```python
from build123d import *

# Parameters (mm, degrees)
F0_R     = 90.4875
F1_DEPTH = 63.5


with BuildPart() as f1:
    # F0 (on Top) → F1 (new body)
    with BuildSketch(Plane.XY):
        Circle(F0_R)
        with BuildLine():
            ThreePointArc((-6.35, -88.672924), (-76.989658, -44.45), (-79.968005, 38.837201))
            Line((-79.968005, 38.837201), (-77.415028, 37.363239))
            Line((-77.415028, 37.363239), (-74.240028, 42.8625))
            Line((-74.240028, 42.8625), (-71.065028, 48.361761))
            Line((-71.065028, 48.361761), (-73.618005, 49.835723))
            ThreePointArc((-73.618005, 49.835723), (0, 88.9), (73.618005, 49.835723))
            Line((73.618005, 49.835723), (71.065028, 48.361761))
            Line((71.065028, 48.361761), (74.240028, 42.8625))
            Line((74.240028, 42.8625), (77.415028, 37.363239))
            Line((77.415028, 37.363239), (79.968005, 38.837201))
            ThreePointArc((79.968005, 38.837201), (76.989658, -44.45), (6.35, -88.672924))
            Line((6.35, -88.672924), (6.35, -85.725))
            Line((6.35, -85.725), (0, -85.725))
            Line((0, -85.725), (-6.35, -85.725))
            Line((-6.35, -85.725), (-6.35, -88.672924))
        make_face(mode=Mode.SUBTRACT)
    extrude(amount=F1_DEPTH)


solid = f1.part
```
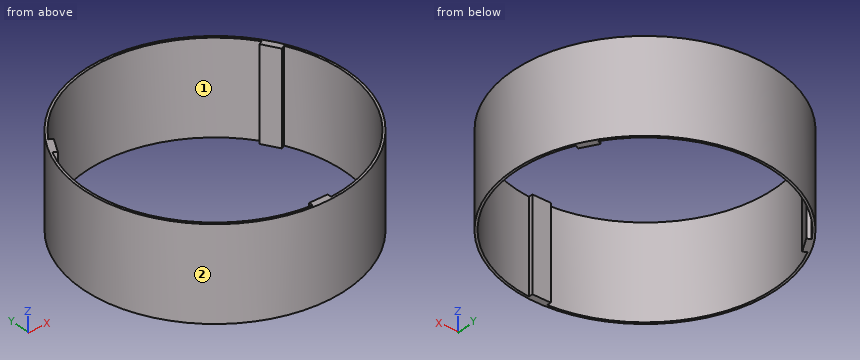
For this review, take the finished solid that the model builds, in its own axes (mm). Face numbers are marked on the shaded views. Round coordinates to 2 decimals unless told otherwise and drop trailing zeros. Write each loop counter-clockwise with the first axis right and the second up, starting at its lowest first coordinate (ties: lowest second). Pieces come first, ordered by that corner, then holes. Notation, with made-up numbers: (-25, 1) -> (22, 1) arc R19 cw to (22, 32) -> close; hole circle Ø4 at (-29, 54). An arc over 180 degrees is marked (long way). One line per question, with ' | ' between items. Start each with the question number.
(1) Add section A-A, the plane x = 0. Write out the cut boundary in (y, z) (1 decimal), plus the area to 3 significant figures.
(2) Add section B-B, the plane y = 0. Write out the cut boundary in (x, z).
(3) Insertion check: P1, Ø3, axis at x = 39.5, z = 9, coming from the +Y side; P2, Ø3, axis at y = 6.5, z = 36, coming from the +X side; P3, Ø8, axis at x = -14.5, z = 40, coming from the -Y side. Each pin has a flat end and moves straight along its axis. Give the tip position at first contact, or say it passes through.
(4) Mouldability with a two-part tool opening along X and no side actions: class the marked faces 1 and 2 as released by +X, released by -X, zero draft, split by the parting line, or undercut.
(5) For line 1 along Y through (x, z) = (0, 17) (1 decimal); line 2 along Y through (x, z) = (-35, 23); line 3 along X through (y, z) = (40, 41), list the stretches that pass through material, from the lowest coordinate up. Write a range as from..to.
Answer list:
1) outline: (-90.5, 0) -> (-85.7, 0) -> (-85.7, 63.5) -> (-90.5, 63.5) -> close; (88.9, 0) -> (90.5, 0) -> (90.5, 63.5) -> (88.9, 63.5) -> close | area: 403 mm²
2) outline: (-90.49, 0) -> (-88.9, 0) -> (-88.9, 63.5) -> (-90.49, 63.5) -> close; (88.9, 0) -> (90.49, 0) -> (90.49, 63.5) -> (88.9, 63.5) -> close
3) P1: y = 82.12 | P2: x = 90.35 | P3: y = -89.88
4) face 1: undercut | face 2: split by the parting line
5) line 1: -90.5..-85.7, 88.9..90.5 | line 2: -83.44..-81.72, 81.72..83.44 | line 3: -81.17..-75.89, 75.89..81.17
